```python
from build123d import *

# Parameters (mm, degrees)
ESQUISSE1_W             = 39
ESQUISSE1_H             = 17
BOSS_EXTRU_1_DEPTH      = 1.5
BOSS_EXTRU_2_DEPTH      = 6
ESQUISSE2_R             = 1.5
ENL_V_MAT_EXTRU_1_DEPTH = 13
CHANFREIN1_SIZE         = 1.5
ESQUISSE4_W             = 7
ESQUISSE4_H             = 15
BOSS_EXTRU_3_DEPTH      = 10
CHANFREIN2_SIZE         = 3
CHANFREIN2_SIZE2        = 1.732050808
CHANFREIN2_PART_2_SIZE  = 3
CHANFREIN2_PART_2_SIZE2 = 1.732050808


with BuildPart() as part:
    # Esquisse1 → Boss.-Extru.1 (new body)
    with BuildSketch(Plane.XY):
        Rectangle(ESQUISSE1_W, ESQUISSE1_H)
    extrude(amount=BOSS_EXTRU_1_DEPTH)

    # Esquisse3 → Boss.-Extru.2 (add)
    with BuildSketch(Plane(origin=(0, -8.5, 0), x_dir=(1, 0, 0), z_dir=(0, 1, 0))):
        Polygon((19.5, 0), (19.5, 3), (12.5, 3), (12.5, 10.5), (8.5, 10.5), (8.5, 3), (5.5, 3), (5.5, 10.5), (1.5, 10.5), (1.5, 3), (-5.5, 3), (-5.5, 0), align=None)
    extrude(amount=BOSS_EXTRU_2_DEPTH)

    # Esquisse2 → Enlèv. mat.-Extru.1 (cut, through all)
    with BuildSketch(Plane.XY.offset(1.5)):
        with Locations((16.5, -5.5)):
            Circle(ESQUISSE2_R)
        with Locations((-3.5, -5.5)):
            Circle(ESQUISSE2_R)
    extrude(amount=-ENL_V_MAT_EXTRU_1_DEPTH, mode=Mode.SUBTRACT)

    # Chanfrein1
    chanfrein1_edges = [part.edges().sort_by_distance(p)[0] for p in [
        (12.5, -5.5, -10.5),
    ]]
    chamfer(chanfrein1_edges, length=CHANFREIN1_SIZE)

    # Esquisse4 → Boss.-Extru.3 (add)
    with BuildSketch(Plane(origin=(0, 0, 0), x_dir=(-1, 0, 0), z_dir=(0, 0, -1))):
        with Locations((15.534193906, 0)):
            Rectangle(ESQUISSE4_W, ESQUISSE4_H)
    extrude(amount=BOSS_EXTRU_3_DEPTH)

    # Chanfrein2
    chanfrein2_edges = [part.edges().sort_by_distance(p)[0] for p in [
        (-12.034193906, 0, -10),
    ]]
    chanfrein2_side = [part.faces().sort_by_distance(p)[0] for p in [
        (-12.034193906, 0, -5),
    ]]
    chamfer(chanfrein2_edges, length=CHANFREIN2_SIZE, length2=CHANFREIN2_SIZE2, reference=chanfrein2_side[0])

    # Chanfrein2 part 2
    chanfrein2_part_2_edges = [part.edges().sort_by_distance(p)[0] for p in [
        (-19.034193906, 0, -10),
    ]]
    chanfrein2_part_2_side = [part.faces().sort_by_distance(p)[0] for p in [
        (-19.034193906, 0, -5),
    ]]
    chamfer(chanfrein2_part_2_edges, length=CHANFREIN2_PART_2_SIZE, length2=CHANFREIN2_PART_2_SIZE2, reference=chanfrein2_part_2_side[0])


solid = part.part
```
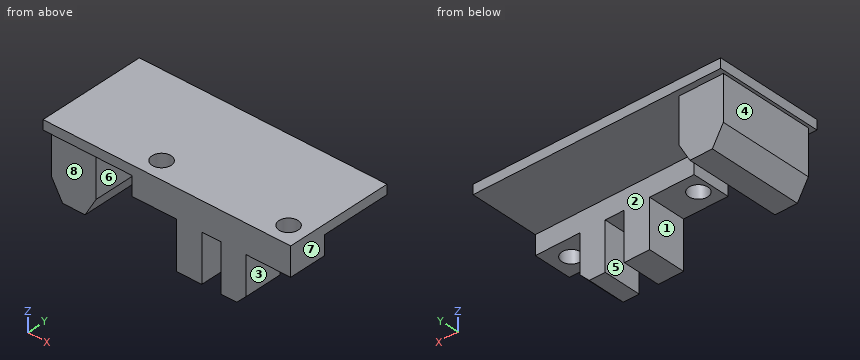
For this review, take the finished solid that the model builds, in its own axes (mm). Face numbers are marked on the shaded views. A direction names the side the tool comes from. Round coordinates to 2 decimals unless told otherwise and drop trailing zeros. Write each loop counter-clockwise with the first axis right and the second up, starting at its lowest first coordinate (ties: lowest second). Pieces come first, ordered by that corner, then holes.
1) Take a section at C-C on z = -4.5. Give the boundary of the cut face in (x, y).
Answer below:
outline: (-19.03, -7.5) - (-12.03, -7.5) - (-12.03, 7.5) - (-19.03, 7.5) - close; (1.5, -8.5) - (5.5, -8.5) - (5.5, -2.5) - (1.5, -2.5) - close; (8.5, -8.5) - (12.5, -8.5) - (12.5, -2.5) - (8.5, -2.5) - close
2) Take a section at B-B on x = -3.5. Give the boundary of the cut face in (y, z).
Answer below:
outline: (-8.5, -3) - (-7, -3) - (-7, 1.5) - (-8.5, 1.5) - close; (-4, -3) - (-2.5, -3) - (-2.5, 0) - (8.5, 0) - (8.5, 1.5) - (-4, 1.5) - close
3) For line 1 along Y through (x, z) = (-3.5, 0.4); line 2 along X through (y, z) = (-7.25, -4.75); line 3 along Y through (x, z) = (-3.5, -1.1), list the stretches that pass through material, from the lowest coordinate up.
Answer below:
line 1: y = -8.5 to -7, -4 to 8.5
line 2: x = -19.03 to -12.03, 1.5 to 5.5, 8.5 to 12.5
line 3: y = -8.5 to -7, -4 to -2.5
4) Insertion check: pin 1 Ø3.5 at (y, z) = (-2, -4) entering from +X; pin 2 Ø3.5 at (y, z) = (-3, -2) entering from -X; pin 3 Ø5.5 at (x, z) = (-16, -7) entering from +Y; pin 4 Ø1.8 at (x, y) = (-15, 2) entering from -Z. Each pin has a flat end and moves straight along its axis. Give the tip position at first contact, or say it passes through.
Answer below:
pin 1: stops at x = 19.5
pin 2: stops at x = -19.03
pin 3: stops at y = 7.5
pin 4: stops at z = -10
5) Take a section at A-A on y = -5.5. State how many separate pieces and enclosed holes the cut face has, then the cut area to 3 significant figures.
Answer below:
separate pieces: 3
enclosed holes: 0
area: 230 mm2
6) Mouldability with a two-part tool opening along X and no side actions: class the marked faces 5, 6, 7 and 8 as +X half, -X half, draft (parallel to the pull), parting line (faces both ways), or undercut.
Answer below:
face 5: undercut
face 6: undercut
face 7: +X half
face 8: draft
7) Machinability: for the marked faces 1, 2, 3 and 4, which of the approach directions +Z, -Z, +X, -X, +Y, -Y give a long, thin tool a straight path to every point of the face, cutting with its end or side? Answer none if there is none.
Answer below:
face 1: -Z, +Y, -Y
face 2: -Z, +X, +Y
face 3: -Z, +X, +Y, -Y
face 4: -Z, -X, +Y, -Y
8) Take a section at D-D on y = 0. Give the boundary of the cut face in (x, z).
Answer below:
outline: (-19.5, 0) - (-19.03, 0) - (-19.03, -7) - (-17.3, -10) - (-13.77, -10) - (-12.03, -7) - (-12.03, 0) - (19.5, 0) - (19.5, 1.5) - (-19.5, 1.5) - close
